Could you check a few things on this model? Use its own coordinates, in mm. A direction names the side the tool comes from. Coordinates: 2 decimals unless noted, no trailing zeros. Order: outer loops, then holes, each group sorted by start corner. A loop starts at its lowest first (then second) coordinate and runs counter-clockwise, first axis right, second up. Notation, with made-up numbers: (72.25, 32.25) - (81.25, 32.25) arc R14 ccw to (81.25, 53.25) - close; hole circle Ø7 at (17.25, 81). An arc over 180 degrees is marked (long way). Answer as CSV lines item,"result". Start each with the question number.
1. I need wall thicknesses on probe 1 along Y at (x, z) = (0, 2.5); probe 2 along X at (y, z) = (-34.5, 15); probe 3 along Z at (x, y) = (50.5, -30). Which ranges of each line are inside material? Lowest first, please.
2. I want a section at C-C, the plane y = 0. List the corners of the cut face in (x, z) for me, and give its area (3 significant figures).
3. I want a section at B-B, the plane z = 26. List the corners of the cut face in (x, y) for me, and give its area (3 significant figures).
4. For faces 1 (the face through (101.873, 1, 27)), 2 (the face through (15, -20, 6)), 3 (the face through (113.873, 1, 21)), 4 (the face through (55.789, 36.483, 39.93)), 5 (the face through (15, 20, 6)), which set-ups out of +Z, -Z, +X, -X, +Y, -Y let a thin tool reach every point of the face, with its end or its side?
5. I want a section at A-A, the plane y = 24. List the corners of the cut face in (x, z) for me.
6. Thinking about a two-plate mould opening in X: for faces 6 (the face through (70.217, -19.262, 5.916)), 7 (the face through (107.789, -39.514, 39.666)), 8 (the face through (-20, 0, 6)), which applies, released by +X, released by -X, zero draft, split by the parting line, or undercut?
7. For pin 1 (3 mm diameter, centred on x = 13.5, y = 9, fed in from +Z); pin 2 (12 mm diameter, centred on y = 15.5, z = 6, fed in from -X); pin 3 (9.5 mm diameter, centred on x = 15, z = 4, fed in from -Y); pin 4 (6 mm diameter, centred on x = 75.21, y = 14.52, fed in from -Z), each with a flat end and sliding along its axis, tell me the tip position at first contact or that it passes through.
8. I want a section at D-D, the plane z = 41.5. List the corners of the cut face in (x, y) for me.
from build123d import *

# Parameters (mm, degrees)
F0_R     = 5
F0_R_2   = 6
F1_DEPTH = 12
F3_DEPTH = 80
F4_R     = 7
F5_W     = 64
F5_H     = 12
F6_DEPTH = 77.1


with BuildPart() as f1:
    # F0 (on Top) → F1 (new body)
    with BuildSketch(Plane.XY):
        with BuildLine():
            Line((29.965228, 20), (0, 20))
            ThreePointArc((0, 20), (-20, 0), (0, -20))
            Line((0, -20), (29.860913, -20))
            ThreePointArc((29.860913, -20), (44.003049, -25.857864), (49.860913, -40))
            Line((49.860913, -40), (102, -40))
            Line((102, -40), (102, -33))
            Line((102, -33), (113.873083, -33))
            Line((113.873083, -33), (113.873083, 33))
            Line((113.873083, 33), (102, 33))
            Line((102, 33), (102, 40))
            Line((102, 40), (50, 40))
            ThreePointArc((50, 40), (44.142136, 25.857864), (30, 20))
            Line((30, 20), (29.965228, 20))
        make_face()
        with Locations((75.211979, -19.481467)):
            Circle(F0_R, mode=Mode.SUBTRACT)
        Circle(F0_R_2, mode=Mode.SUBTRACT)
        with Locations((75.211979, 14.518533)):
            Circle(F0_R, mode=Mode.SUBTRACT)
    extrude(amount=F1_DEPTH)

    # F2 (on face) → F3 (join)
    with BuildSketch(Plane(origin=(0, 40, 0), x_dir=(-1, 0, 0), z_dir=(0, 1, 0))):
        Polygon((-113.873083, 52), (-113.873083, 0), (-102, 0), (-102, 12), (-101.873083, 12), (-101.873083, 52), align=None)
        Polygon((-61.873083, 52), (-61.873083, 12), (-50, 12), (-50, 0), (-49.873083, 0), (-49.873083, 52), align=None)
    extrude(amount=-F3_DEPTH)

    # F4
    f4_edges = [f1.edges().sort_by_distance(p)[0] for p in [
        (107.873083, 40, 52),
        (55.873083, 40, 52),
        (55.873083, -40, 52),
        (107.873083, -40, 52),
        (61.873083, 0, 52),
    ]]
    fillet(f4_edges, radius=F4_R)

    # F5 (on face) → F6 (cut)
    with BuildSketch(Plane(origin=(49.873083, 0, 0), x_dir=(0, -1, 0), z_dir=(-1, 0, 0))):
        with Locations((1.51522, 39.79838)):
            Rectangle(F5_W, F5_H)
        with BuildLine():
            Line((-30.48478, 33.79838), (-30.48478, 45.79838))
            ThreePointArc((-30.48478, 45.79838), (-36.48478, 39.79838), (-30.48478, 33.79838))
        make_face()
        with BuildLine():
            ThreePointArc((33.51522, 33.79838), (39.51522, 39.79838), (33.51522, 45.79838))
            Line((33.51522, 45.79838), (33.51522, 33.79838))
        make_face()
    extrude(amount=-F6_DEPTH, mode=Mode.SUBTRACT)


solid = f1.part
Solved:
1,probe 1,"y = -20 to -6, 6 to 20"
1,probe 2,"x = 49.87 to 61.87, 101.87 to 113.87"
1,probe 3,"z = 0 to 33.8, 45.8 to 52"
2,outline,"(-20, 0) - (-6, 0) - (-6, 12) - (-20, 12) - close; (6, 0) - (113.87, 0) - (113.87, 33.8) - (101.87, 33.8) - (101.87, 12) - (61.87, 12) - (61.87, 33.8) - (49.87, 33.8) - (49.87, 12) - (6, 12) - close; (49.87, 45.8) - (61.83, 45.8) arc R7 ccw to (54.87, 52) - (49.87, 52) - close; (101.87, 45.8) - (113.87, 45.8) - (113.87, 52) - (101.87, 52) - close"
2,area,"2,120 mm2"
3,outline,"(49.87, -40) - (61.87, -40) - (61.87, 40) - (49.87, 40) - close; (101.87, -40) - (113.87, -40) - (113.87, 40) - (101.87, 40) - close"
3,area,"1,920 mm2"
4,face 1,"+Z, +Y, -Y"
4,face 2,"+Z, -Z, -X, -Y"
4,face 3,"+Z, -Z, +X, +Y, -Y"
4,face 4,"+X, -X"
4,face 5,"+Z, -Z, -X, +Y"
5,outline,"(42, 0) - (113.87, 0) - (113.87, 33.8) - (101.87, 33.8) - (101.87, 12) - (61.87, 12) - (61.87, 33.8) - (49.87, 33.8) - (49.87, 12) - (42, 12) - close; (49.87, 45.8) - (61.83, 45.8) arc R7 ccw to (54.87, 52) - (49.87, 52) - close; (101.87, 45.8) - (113.87, 45.8) - (113.87, 52) - (101.87, 52) - close"
6,face 6,"undercut"
6,face 7,"zero draft"
6,face 8,"released by -X"
7,pin 1,"stops at z = 12"
7,pin 2,"stops at x = -17.6"
7,pin 3,"stops at y = -20"
7,pin 4,"passes through"
8,outline,"(49.87, -40) - (61.87, -40) - (61.87, -39.27) - (49.87, -39.27) - close; (49.87, 36.24) - (61.87, 36.24) - (61.87, 40) - (49.87, 40) - close; (101.87, -40) - (113.87, -40) - (113.87, -39.27) - (101.87, -39.27) - close; (101.87, 36.24) - (113.87, 36.24) - (113.87, 40) - (101.87, 40) - close"
